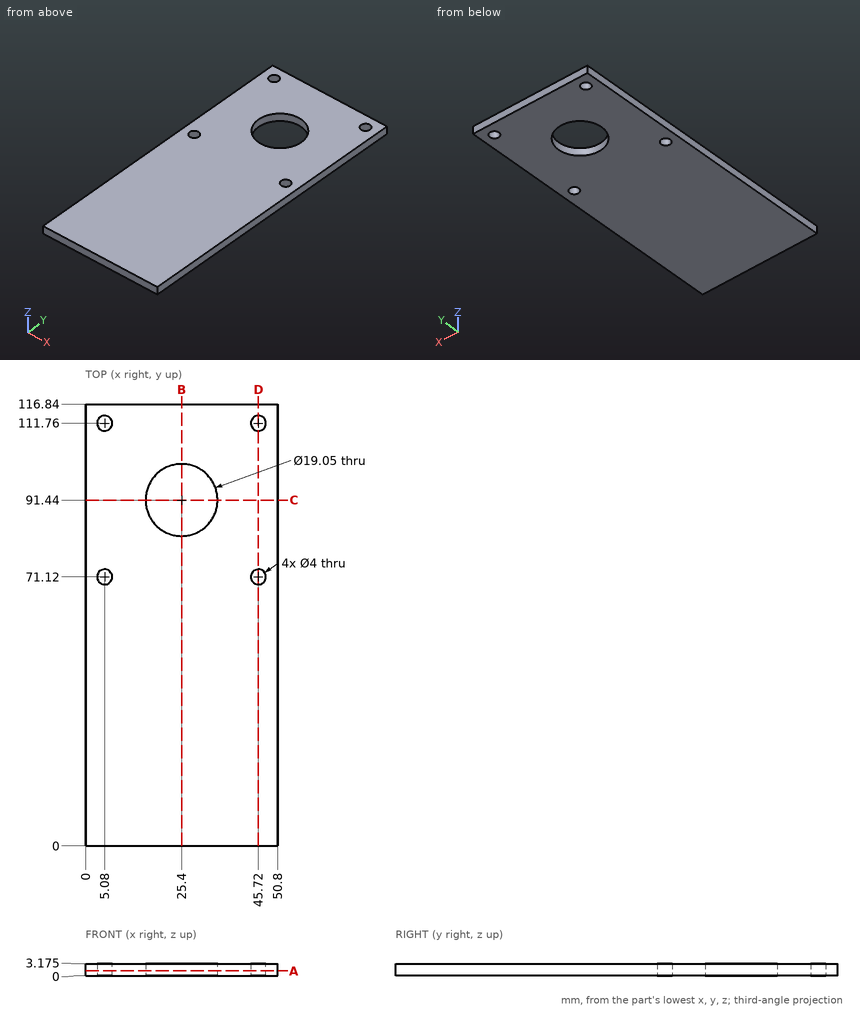
Job drawing, mm, ordinate dimensions from the low corner. One solid piece. Give positions to 0.01 mm unless a question says otherwise; leave off trailing zeros. Loops run counter-clockwise (first coordinate to the right, second up) from the corner with the lowest first, then second, coordinate; pieces in that order, holes last. Notation, with made-up numbers: M 72,24.5 L 102,24.5 A21 cw 102,28.5 Z; hole C 15.25,-2 d6. An arc over 180 degrees is marked long. Return JSON: item names as keys, results as strings.
1) Saw through at C-C, the plane y = 91.44. List the corners of the cut face in (x, z) (3 decimals), then the cut area to 3 significant figures.
Calculated:
{"outline": "M 0,0 L 15.875,0 L 15.875,3.175 L 0,3.175 Z; M 34.925,0 L 50.8,0 L 50.8,3.175 L 34.925,3.175 Z", "area": "101 mm2"}
2) Drill centre lines: line 1 (Y direction, x = 5.08, z = 1.3); line 2 (Y direction, x = 25, z = 2.55); line 3 (Y direction, x = 46.5, z = 1.4). Where is each one in solid material? Low to high.
Calculated:
{"line 1": "y = 0 to 69.12, 73.12 to 109.76, 113.76 to 116.84", "line 2": "y = 0 to 81.92, 100.96 to 116.84", "line 3": "y = 0 to 69.28, 72.96 to 109.92, 113.6 to 116.84"}
3) Saw through at B-B, the plane x = 25.4. List the corners of the cut face in (y, z) (3 decimals).
Calculated:
{"outline": "M 0,0 L 81.915,0 L 81.915,3.175 L 0,3.175 Z; M 100.965,0 L 116.84,0 L 116.84,3.175 L 100.965,3.175 Z"}
4) Saw through at A-A, the plane z = 1.3. List the corners of the cut face in (x, y) (3 decimals).
Calculated:
{"outline": "M 0,0 L 50.8,0 L 50.8,116.84 L 0,116.84 Z; hole C 5.08,71.12 d4; hole C 5.08,111.76 d4; hole C 25.4,91.44 d19.05; hole C 45.72,71.12 d4; hole C 45.72,111.76 d4"}
5) Saw through at D-D, the plane x = 45.72. List the corners of the cut face in (y, z) (3 decimals), then the cut area to 3 significant figures.
Calculated:
{"outline": "M 0,0 L 69.12,0 L 69.12,3.175 L 0,3.175 Z; M 73.12,0 L 109.76,0 L 109.76,3.175 L 73.12,3.175 Z; M 113.76,0 L 116.84,0 L 116.84,3.175 L 113.76,3.175 Z", "area": "346 mm2"}
